Input: dimensioned drawing with shaded views. Units: mm. Origin: part minimum x, y, z. A direction names the side the tool comes from. Coordinates: 2 decimals unless noted, no trailing zeros. Loops run counter-clockwise (first coordinate to the right, second up) from the corner with the lowest first, then second, coordinate; pieces in that order, holes last. Notation, with made-up numbers: (-27.5, 45) - (30.5, 45) arc R30 cw to (30.5, 76) - close; hole circle Ø8 at (66.25, 63). An arc over 180 degrees is marked (long way). Put each result on its own line as item: value. Start each with the question number.
1) Contact query for flat-ended pins moving along their axis: pin 1 Ø12 at (y, z) = (64, 16) entering from +X; pin 2 Ø4 at (x, y) = (70.5, 69.5) entering from +Z. Output: stop coordinate, or through.
2) Material intervals for line 1 along Y through (x, z) = (36, 36); line 2 along X through (y, z) = (95.5, 66); line 3 along Y through (x, z) = (11, 72.5), sorted ascending. Write a range as from..to.
3) Section C-C on y = 56. Output: boundary loops of the cut face in (x, z).
4) Section D-D on y = 15. Output: boundary loops of the cut face in (x, z).
5) Draft query along Y for the marked faces 1, 2 and 3. Return one class per face: +Y half, -Y half, draft (parallel to the pull), parting line (faces both ways), or undercut.
6) Reachability of the marked faces 4, 5, 6, 7 and 8 from +Z, -Z, +X, -X, +Y, -Y: full face, straight path, thin tool, end or side. Return the list, or none.
7) Section A-A on z = 31. Output: boundary loops of the cut face in (x, y), and give its area (3 significant figures).
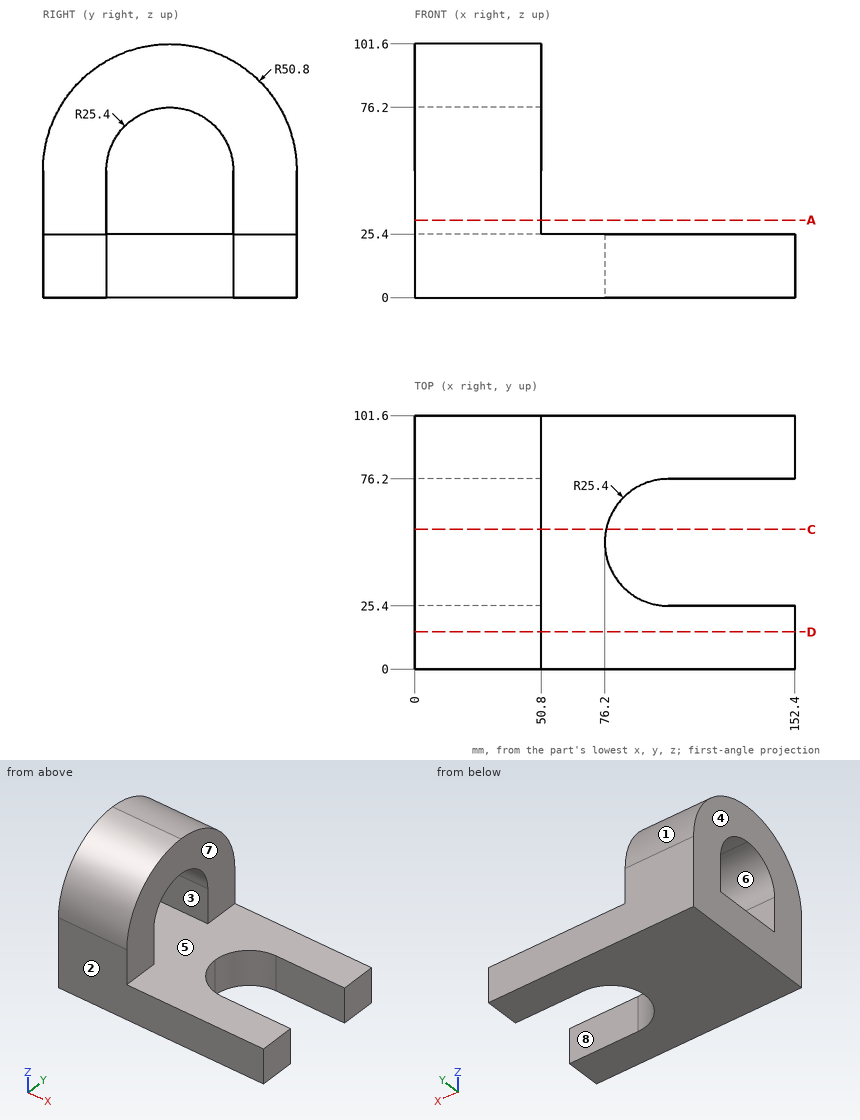
Answer block:
1. pin 1: stops at x = 84.97
1. pin 2: stops at z = 25.4
2. line 1: y = 0..25.4, 76.2..101.6
2. line 2: x = 0..50.8
2. line 3: y = 4.87..37.6, 64..96.73
3. outline: (0, 0) - (76.74, 0) - (76.74, 25.4) - (0, 25.4) - close; (0, 75.66) - (50.8, 75.66) - (50.8, 101.33) - (0, 101.33) - close
4. outline: (0, 0) - (152.4, 0) - (152.4, 25.4) - (50.8, 25.4) - (50.8, 86.84) - (0, 86.84) - close
5. face 1: +Y half
5. face 2: -Y half
5. face 3: undercut
6. face 4: +Z, -Z, -X, +Y, -Y
6. face 5: +X
6. face 6: +X, -X
6. face 7: +Z, +X, +Y, -Y
6. face 8: +Z, -Z, +X
7. outline: (0, 0) - (50.8, 0) - (50.8, 25.4) - (0, 25.4) - close; (0, 76.2) - (50.8, 76.2) - (50.8, 101.6) - (0, 101.6) - close
7. area: 2,580 mm²
